from build123d import *

# Parameters (mm, degrees)
SKETCH1_R           = 70.952762223
SKETCH1_R_2         = 60
BOSS_EXTRUDE1_DEPTH = 20


with BuildPart() as part:
    # Sketch1 → Boss-Extrude1 (new, symmetric)
    # profile 1 of 2: a face of its own
    with BuildSketch(Plane.XY):
        with BuildLine():
            Line((40.505236387, 90.426645724), (-25.752991774, 90.426645724))
            ThreePointArc((-25.752991774, 90.426645724), (-80.41932051, 36.078066751), (-74.051220561, -40.74395377))
            ThreePointArc((-74.051220561, -40.74395377), (-42.820207747, -72.228243513), (0, -83.763687608))
            ThreePointArc((0, -83.763687608), (55.05134178, -58.365548869), (71.457998611, 0))
            ThreePointArc((71.457998611, 0), (-63.58670667, -30.438746727), (45.341543852, 54.990908339))
            Line((45.341543852, 54.990908339), (72.624781189, 54.990908339))
            Line((72.624781189, 54.990908339), (72.624781189, 90.426645724))
            Line((72.624781189, 90.426645724), (40.505236387, 90.426645724))
        make_face()
    # profile 2 of 2: a face of its own
    with BuildSketch(Plane.XY):
        with Locations((0.505236387, 0)):
            Circle(SKETCH1_R)
        with Locations((-0.148485531, 0.959241536)):
            Circle(SKETCH1_R_2, mode=Mode.SUBTRACT)
    extrude(amount=BOSS_EXTRUDE1_DEPTH, both=True)


solid = part.part
Here's how the part is built. I have some questions about the finished solid (model axes, mm). Round coordinates to 2 decimals unless told otherwise and drop trailing zeros. Loops run counter-clockwise (first coordinate to the right, second up) from the corner with the lowest first, then second, coordinate; pieces in that order, holes last. Notation, with made-up numbers: (-20, 10) -> (7, 10) arc R14 cw to (7, 15) -> close; hole circle Ø4 at (-33.75, 85). An arc over 180 degrees is marked (long way). Write each question's results on one line, items separated by ' | '.
(1) If I drill on L1, parallel to Y at x = 2, z = 11; L2, parallel to Y at x = 10, z = -14; L3, parallel to X at y = 29, z = 13.5, over which ranges is the centre line in solid material (lowest first)?
Worked answers:
L1: -83.74 to -59, 60.92 to 90.43 | L2: -83.07 to -58.18, 60.09 to 90.43 | L3: -82.7 to -53.19, 52.9 to 65.26
(2) If we section it at A-A, the plane x = -48: List the corners of the cut face in (y, z) for me.
Worked answers:
outline: (-68.96, -20) -> (-35.24, -20) -> (-35.24, 20) -> (-68.96, 20) -> close; (37.16, -20) -> (78.7, -20) -> (78.7, 20) -> (37.16, 20) -> close
(3) If we section it at B-B, the plane y = -28: List the corners of the cut face in (x, z) for me, then the cut area to 3 significant figures.
Worked answers:
outline: (-80.07, -20) -> (-52.7, -20) -> (-52.7, 20) -> (-80.07, 20) -> close; (52.4, -20) -> (70.43, -20) -> (70.43, 20) -> (52.4, 20) -> close | area: 1,820 mm2
(4) For P1, Ø2, axis at x = 43, z = 0.5, coming from the -Y side; P2, Ø3, axis at x = -62, z = -15, coming from the -Y side; P3, Ø1, axis at y = 41, z = 1, coming from the -X side, each with a flat end and sliding along its axis, tell me the tip position at first contact or that it passes through.
Worked answers:
P1: y = -70.33 | P2: y = -58.57 | P3: x = -78.66
(5) If we section it at C-C, the plane x = 54: List the corners of the cut face in (y, z) for me.
Worked answers:
outline: (-59.57, -20) -> (-24.89, -20) -> (-24.89, 20) -> (-59.57, 20) -> close; (26.8, -20) -> (46.61, -20) -> (46.61, 20) -> (26.8, 20) -> close; (54.99, -20) -> (90.43, -20) -> (90.43, 20) -> (54.99, 20) -> close
(6) If we section it at D-D, the plane z = 3.5: List the corners of the cut face in (x, y) for me, then the cut area to 3 significant figures.
Worked answers:
outline: (-74.05, -40.74) arc R85.24 ccw to (0, -83.76) arc R72.36 ccw to (71.46, 0) arc R70.95 ccw to (45.34, 54.99) -> (72.62, 54.99) -> (72.62, 90.43) -> (-25.75, 90.43) arc R91.36 ccw to start; hole circle Ø120 at (-0.15, 0.96) | area: 11,700 mm2
